Work out the finished part from the listing and answer in its coordinate system (mm). Face numbers are marked on the shaded views. A direction names the side the tool comes from. Round coordinates to 2 decimals unless told otherwise and drop trailing zeros. Order: outer loops, then holes, each group sorted by start corner. A loop starts at its lowest first (then second) coordinate and runs counter-clockwise, first axis right, second up. Notation, with made-up numbers: (83, -25) - (104, -25) arc R23 cw to (104, -13) - close; hole circle Ø5 at (-11.75, -38.75). An arc over 180 degrees is marked (long way). Answer in a Markdown table with one row per item.
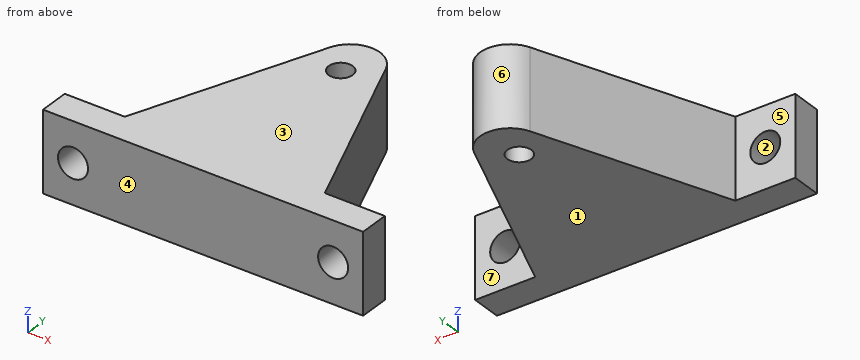
from build123d import *

# Parameters (mm, degrees)
ESQUISSE1_R             = 1.2
BOSS_EXTRU_1_DEPTH      = 8
ESQUISSE2_R             = 1.5
ENL_V_MAT_EXTRU_1_DEPTH = 39.721703123


with BuildPart() as part:
    # Esquisse1 → Boss.-Extru.1 (new body)
    with BuildSketch(Plane.XY):
        with BuildLine():
            Line((0, 0), (32, 0))
            Line((32, 0), (32, 3))
            Line((32, 3), (26, 3))
            Line((26, 3), (18.792908921, 21.37755528))
            ThreePointArc((18.792908921, 21.37755528), (16, 23.282265473), (13.207091079, 21.37755528))
            Line((13.207091079, 21.37755528), (6, 3))
            Line((6, 3), (0, 3))
            Line((0, 3), (0, 0))
        make_face()
        with Locations((16, 19)):
            Circle(ESQUISSE1_R, mode=Mode.SUBTRACT)
    extrude(amount=BOSS_EXTRU_1_DEPTH)

    # Esquisse2 → Enlèv. mat.-Extru.1 (cut, through all)
    with BuildSketch(Plane(origin=(0, 3, 0), x_dir=(1, 0, 0), z_dir=(0, 1, 0))):
        with Locations(Location((3, -4, 0), (0, 0, 180))):
            Circle(ESQUISSE2_R)
        with Locations((29, -4)):
            Circle(ESQUISSE2_R)
    extrude(amount=-ENL_V_MAT_EXTRU_1_DEPTH, mode=Mode.SUBTRACT)


solid = part.part
1) Find section D-D, the plane y = 19. Give the vertices of the cut face in (x, z), then the cut area to 3 significant figures.
Filled in:
| item | result |
|---|---|
| outline | (12.27, 0) - (14.8, 0) - (14.8, 8) - (12.27, 8) - close; (17.2, 0) - (19.73, 0) - (19.73, 8) - (17.2, 8) - close |
| area | 40.4 mm^2 |
2) Find section C-C, the plane z = 7. Give the vertices of the cut face in (x, y).
Filled in:
| item | result |
|---|---|
| outline | (0, 0) - (32, 0) - (32, 3) - (26, 3) - (18.79, 21.38) arc R3 ccw to (13.21, 21.38) - (6, 3) - (0, 3) - close; hole circle Ø2.4 at (16, 19) |
3) The mould has two halves that part along Z. Classify the marked faces 1, 2, 3 and 4: released by +Z, released by -Z, zero draft, split by the parting line, or undercut.
Filled in:
| item | result |
|---|---|
| face 1 | released by -Z |
| face 2 | undercut |
| face 3 | released by +Z |
| face 4 | zero draft |
4) Find section B-B, the plane x = 29. Give the vertices of the cut face in (y, z).
Filled in:
| item | result |
|---|---|
| outline | (0, 0) - (3, 0) - (3, 2.5) - (0, 2.5) - close; (0, 5.5) - (3, 5.5) - (3, 8) - (0, 8) - close |
5) Find section A-A, the plane z = 4. Give the vertices of the cut face in (x, y), then the cut area to 3 significant figures.
Filled in:
| item | result |
|---|---|
| outline | (0, 0) - (1.5, 0) - (1.5, 3) - (0, 3) - close; (4.5, 0) - (27.5, 0) - (27.5, 3) - (26, 3) - (18.79, 21.38) arc R3 ccw to (13.21, 21.38) - (6, 3) - (4.5, 3) - close; (30.5, 0) - (32, 0) - (32, 3) - (30.5, 3) - close; hole circle Ø2.4 at (16, 19) |
| area | 316 mm^2 |
6) Which of the six approach directions +Z, -Z, +X, -X, +Y, -Y give full straight-line access (tool end or side, diameter ignored) to the marked faces 5, 6 and 7?
Filled in:
| item | result |
|---|---|
| face 5 | +Z, -Z, -X, +Y |
| face 6 | +Z, -Z, +Y |
| face 7 | +Z, -Z, +X, +Y |
7) Each of these flat-tipped pins is pushed along its axis until it touches: pin 1 (3 mm diameter, centred on x = 28, z = 2.5, fed in from +Y); pin 2 (8 mm diameter, centred on x = 4.5, y = 12, fed in from -Z); pin 3 (2 mm diameter, centred on y = 18, z = 2, fed in from -X); pin 4 (4 mm diameter, centred on y = 11.5, z = 2, fed in from -X). Where does it stop, or does it pass through?
Filled in:
| item | result |
|---|---|
| pin 1 | stops at y = 3 |
| pin 2 | passes through |
| pin 3 | stops at x = 11.49 |
| pin 4 | stops at x = 8.55 |
8) Find the intervals of material crossed by probe 1 along Z at (x, y) = (29, 2.05); probe 2 along Y at (x, z) = (29.5, 7.25); probe 3 along X at (y, z) = (14.25, 2.5), in increasing order. Write a range as from..to.
Filled in:
| item | result |
|---|---|
| probe 1 | z = 0..2.5, 5.5..8 |
| probe 2 | y = 0..3 |
| probe 3 | x = 10.41..21.59 |
